Source: CAD feature listing. Evaluate the final solid. Frame: model axes, mm. A direction names the side the tool comes from. Give positions to 0.01 mm unless a question says otherwise; leave off trailing zeros. Order: outer loops, then holes, each group sorted by start corner. A loop starts at its lowest first (then second) coordinate and runs counter-clockwise, first axis right, second up.
```python
from build123d import *

# Parameters (mm, degrees)
SCHIZZO1_R                   = 1
ESTRUSIONE_ESTRUSIONE1_DEPTH = 2
SCHIZZO2_W                   = 12
SCHIZZO2_H                   = 7
ESTRUSIONE_ESTRUSIONE2_DEPTH = 1


with BuildPart() as part:
    # Schizzo1 → Estrusione-Estrusione1 (new body)
    with BuildSketch(Plane.XY):
        Polygon((0, 0), (10, 0), (14, 8), (17, 8), (17, 17), (14, 17), align=None)
        with Locations((15.5, 15.5)):
            Circle(SCHIZZO1_R, mode=Mode.SUBTRACT)
        with Locations((15.5, 12.5)):
            Circle(SCHIZZO1_R, mode=Mode.SUBTRACT)
        with Locations((15.5, 9.5)):
            Circle(SCHIZZO1_R, mode=Mode.SUBTRACT)
    extrude(amount=ESTRUSIONE_ESTRUSIONE1_DEPTH)

    # Schizzo2 → Estrusione-Estrusione2 (add)
    with BuildSketch(Plane.XZ):
        with Locations((5, 1)):
            Rectangle(SCHIZZO2_W, SCHIZZO2_H)
    extrude(amount=ESTRUSIONE_ESTRUSIONE2_DEPTH)


solid = part.part
```
1) Section query B-B, the plane y = 10. Return the cut outline in (x, z).
Report:
outline: (8.24, 0) - (14.63, 0) - (14.63, 2) - (8.24, 2) - close; (16.37, 0) - (17, 0) - (17, 2) - (16.37, 2) - close
2) Section query C-C, the plane z = 1.25. Return the cut outline in (x, y).
Report:
outline: (-1, -1) - (11, -1) - (11, 0) - (10, 0) - (14, 8) - (17, 8) - (17, 17) - (14, 17) - (0, 0) - (-1, 0) - close; hole circle Ø2 at (15.5, 9.5); hole circle Ø2 at (15.5, 12.5); hole circle Ø2 at (15.5, 15.5)
3) Section query D-D, the plane x = 4.75. Return the cut outline in (y, z), and give its area (3 significant figures).
Report:
outline: (-1, -2.5) - (0, -2.5) - (0, 0) - (5.77, 0) - (5.77, 2) - (0, 2) - (0, 4.5) - (-1, 4.5) - close
area: 18.5 mm2
4) Reachability of faces 4 (the flat face through (15, 8, 1)), 5 (the flat face through (10, 7, 0)), 6 (the flat face through (10, 7, 2)), 7 (the flat face through (7.1, 8.62, 0.99)), 8 (the flat face through (-1, -0.5, 1)) from +Z, -Z, +X, -X, +Y, -Y: full face, straight path, thin tool, end or side. Return the list, or none.
Report:
face 4: +Z, -Z, +X, -Y
face 5: -Z, +X, -X, +Y
face 6: +Z, +X, -X, +Y
face 7: +Z, -Z, -X, +Y
face 8: +Z, -Z, -X, +Y, -Y
5) Pin query (flat end, axial travel): pin 1 (6 mm diameter, centred on x = 10, y = 5.5, fed in from +Z); pin 2 (2 mm diameter, centred on x = 3.5, z = 0.5, fed in from +Y); pin 3 (2.5 mm diameter, centred on x = 15.5, y = 12.5, fed in from -Z). Return the tip coordinate at first contact, or that it passes through.
Report:
pin 1: stops at z = 2
pin 2: stops at y = 5.46
pin 3: stops at z = 0
6) Section query A-A, the plane x = 15.5. Return the cut outline in (y, z), and give its area (3 significant figures).
Report:
outline: (8, 0) - (8.5, 0) - (8.5, 2) - (8, 2) - close; (10.5, 0) - (11.5, 0) - (11.5, 2) - (10.5, 2) - close; (13.5, 0) - (14.5, 0) - (14.5, 2) - (13.5, 2) - close; (16.5, 0) - (17, 0) - (17, 2) - (16.5, 2) - close
area: 6.00 mm2
7) Material intervals for L1, parallel to Y at x = 15.5, z = 0.55; L2, parallel to Z at x = 8, y = 2; L3, parallel to X at y = -0.5, z = 0.75, sorted ascending.
Report:
L1: y = 8 to 8.5, 10.5 to 11.5, 13.5 to 14.5, 16.5 to 17
L2: z = 0 to 2
L3: x = -1 to 11
8) Draft query along Y for faces 1 (the flat face through (11, -0.5, 1)), 2 (the flat face through (5, -1, 1)), 3 (the flat face through (12, 4, 1)). Return one class per face: +Y half, -Y half, draft (parallel to the pull), parting line (faces both ways), or undercut.
Report:
face 1: draft
face 2: -Y half
face 3: undercut
